Can you work these out from the drawing? Everything is in mm from the part's minimum corner. A direction names the side the tool comes from. Round coordinates to 2 decimals unless told otherwise and drop trailing zeros. Write each loop counter-clockwise with the first axis right and the second up, starting at its lowest first coordinate (ties: lowest second). Pieces come first, ordered by that corner, then holes. Notation, with made-up numbers: (12.25, -13.5) -> (24.25, -13.5) arc R26 ccw to (24.25, 6.5) -> close; hole circle Ø5 at (25, 44). An arc over 180 degrees is marked (long way). Put each result on its own line as item: value. Start each with the question number.
1. Which directions (+Z, -Z, +X, -X, +Y, -Y) give clear straight access to the entire face, cutting with the end or side of a thin tool? Please do the marked faces 1 and 2.
2. I need wall thicknesses on probe 1 along X at (y, z) = (18.75, 17.5); probe 2 along Z at (x, y) = (29, 12.75). Which ranges of each line are inside material? Lowest first, please. Write a range as from..to.
3. Suppose I cut it at C-C (x = 43). Please give me the cut outline in (y, z).
4. We'd pull the mould along X, two halves only. Please class the marked faces 3, 4 and 5: +X half, -X half, draft (parallel to the pull), parting line (faces both ways), or undercut.
5. Suppose I cut it at A-A (z = 19). Please give me the cut outline in (x, y).
6. For pin 1 (6 mm diameter, centred on x = 20.5, y = 16.5, fed in from -Z), with a flat end and sliding along its axis, tell me the tip position at first contact or that it passes through.
7. Suppose I cut it at B-B (y = 1.5). Please give me the cut outline in (x, z).
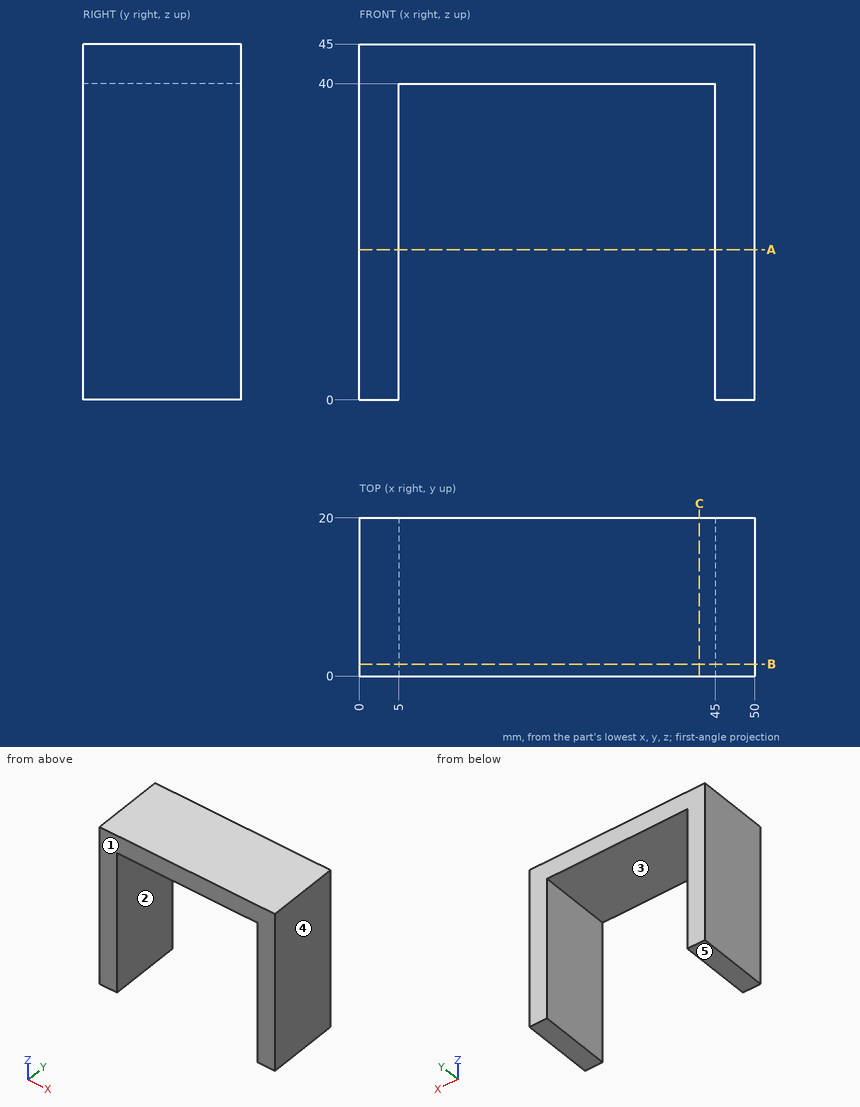
Verdict:
1. face 1: +Z, -Z, +X, -X, -Y
1. face 2: -Z, +Y, -Y
2. probe 1: x = 0..5, 45..50
2. probe 2: z = 40..45
3. outline: (0, 40) -> (20, 40) -> (20, 45) -> (0, 45) -> close
4. face 3: undercut
4. face 4: +X half
4. face 5: draft
5. outline: (0, 0) -> (5, 0) -> (5, 20) -> (0, 20) -> close; (45, 0) -> (50, 0) -> (50, 20) -> (45, 20) -> close
6. pin 1: stops at z = 40
7. outline: (0, 0) -> (5, 0) -> (5, 40) -> (45, 40) -> (45, 0) -> (50, 0) -> (50, 45) -> (0, 45) -> close
